Input: part model. Units: mm. Frame: model coordinates. Face numbers are marked on the shaded views. A direction names the side the tool comes from. Coordinates: 2 decimals unless noted, no trailing zeros. Loops run counter-clockwise (first coordinate to the right, second up) from the corner with the lowest first, then second, coordinate; pieces in that order, holes last. Notation, with made-up numbers: (69.5, -8.75) -> (81.5, -8.75) arc R12 cw to (81.5, 9.25) -> close; hole circle Ø7 at (84.5, -23). An arc over 180 degrees is marked (long way). Put each result on its own line as item: value. Start each with the question number.
1) Contact query for flat-ended pins moving along their axis: P1, Ø2.5, axis at x = 0, z = -45, coming from the +Y side; P2, Ø5, axis at x = -5, z = -47, coming from the -Y side; P3, Ø1.5, axis at y = 9.5, z = -61, coming from the +X side; P4, Ø10.5, axis at x = 7, y = 3.5, coming from the +Z side. Output: stop coordinate, or through.
2) Cut plane D-D (x = 7.5). Return the cut outline in (y, z), plus the area to 3 significant figures.
3) Pull-direction query (X, two-part tool) for the marked faces 1, 2 and 3; classes: pulls with the +X half, pulls with the -X half, needs draft (parallel to the pull), parting line crosses it, or undercut.
4) Cut plane C-C (y = 0). Return the cut outline in (x, z).
5) Cut plane A-A (x = 0). State how many separate pieces and enclosed holes the cut face has, plus the area to 3 significant figures.
6) Material intervals for L1, parallel to Z at x = 0, y = -20; L2, parallel to Y at x = 0, z = -43.25; L3, parallel to X at y = 0, z = -55.75, sorted ascending.
7) Set-up query: the marked faces 4 and 5. Return all of +Z, -Z, +X, -X, +Y, -Y with unobstructed straight access to the full face (end or side cutting, diameter ignored); none if empty.
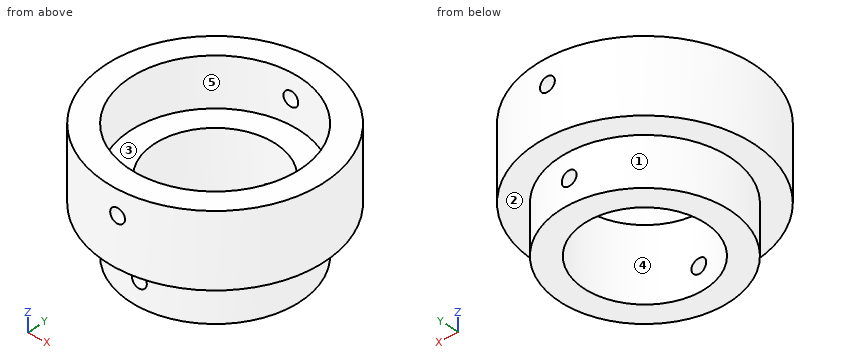
Autodesk Inventor part; units mm, degrees
ref_plane "YZ Plane" through (0, 0, 0) normal (1, 0, 0) x (0, 1, 0)
ref_plane "XZ Plane" through (0, 0, 0) normal (0, 1, 0) x (-1, 0, 0)
ref_plane "XY Plane" through (0, 0, 0) normal (0, 0, 1) x (1, 0, 0)
sketch "Эскиз1" plane through (0, 0, 0) normal (0, 1, 0) x (-1, 0, 0)
  line L0 (17.5, -40) -> (17.5, -50)
  line L1 (17.5, -50) -> (12.5, -50)
  line L2 (12.5, -50) -> (12.5, -65)
  line L3 (12.5, -65) -> (17.5, -65)
  line L4 (22.5, -55) -> (22.5, -40)
  line L5 (22.5, -40) -> (17.5, -40)
  line L6 (12.5, -65) -> (17.5, -65)
  line L7 (22.5, -50) -> (22.5, -55)
  line L8 (22.5, -55) -> (17.5, -55)
  line L9 (17.5, -55) -> (17.5, -65)
  line L10 (12.5, -65) -> (0, -65)
  line L11 (0, -65) -> (0, -40)
  line L12 (17.5, -40) -> (0, -40)
  dimension "d21" = 10
  dimension "d22" = 15
  dimension "d23" = 5
  dimension "d24" = 5
  dimension "d26" = 12.5
  dimension "d39" = 17.5
  dimension "d40" = 5
revolve "Вращение1" add sketch "Эскиз1" angle 360 about axis through (0, 0, -65) along (0, 0, 1) contours L5 L4 L8 L9 L3 L2 L1 L0
sketch "Эскиз4" plane through (0, 0, 0) normal (0, 1, 0) x (-1, 0, 0)
  line L0 (12.5, -65) -> (-12.5, -65)
  line L1 (0, -65) -> (0, -60)
  line L2 (17.5, -40) -> (-17.5, -40)
  line L3 (0, -40) -> (0, -45)
  circle A0 centre (0, -60) radius 1.5
  circle A1 centre (0, -45) radius 1.5
  point P0 (0, 0)
  dimension "d27" = 5
  dimension "d28" = 5
  dimension "d29" = 3
  dimension "d30" = 3
extrude "Выдавливание3" cut sketch "Эскиз4" along normal blind 49.75 and the other way blind 43
thread "Резьба1"
thread "Резьба2"
properties part number "Муфта штурвал, вал 25"
Results found:
1. P1: passes through
1. P2: stops at y = -22.36
1. P3: stops at x = 15.16
1. P4: stops at z = -50
2. outline: (-21.21, -55) -> (-15.81, -55) -> (-15.81, -65) -> (-10, -65) -> (-10, -50) -> (-15.81, -50) -> (-15.81, -40) -> (-21.21, -40) -> close; (10, -65) -> (15.81, -65) -> (15.81, -55) -> (21.21, -55) -> (21.21, -40) -> (15.81, -40) -> (15.81, -50) -> (10, -50) -> close
2. area: 336 mm2
3. face 1: parting line crosses it
3. face 2: needs draft
3. face 3: undercut
4. outline: (-22.5, -55) -> (-17.5, -55) -> (-17.5, -65) -> (-12.5, -65) -> (-12.5, -50) -> (-17.5, -50) -> (-17.5, -40) -> (-22.5, -40) -> close; (12.5, -65) -> (17.5, -65) -> (17.5, -55) -> (22.5, -55) -> (22.5, -40) -> (17.5, -40) -> (17.5, -50) -> (12.5, -50) -> close
5. separate pieces: 6
5. enclosed holes: 0
5. area: 240 mm2
6. L1: z = -55 to -46.5, -43.5 to -40
6. L2: y = -22.5 to -17.5, 17.5 to 22.5
6. L3: x = -17.5 to -12.5, 12.5 to 17.5
7. face 4: +Z, -Z
7. face 5: +Z
